```python
from build123d import *

# Parameters (mm, degrees)
SKETCH1_W                 = 14.2875
SKETCH1_H                 = 6.35
EXTRUDE1_DEPTH            = 44.45
F_6_CLEARANCE_HOLE1_D     = 3.7973
F_6_CLEARANCE_HOLE1_DEPTH = 6.35
F_6_CLEARANCE_HOLE1_TIP   = 1.140824014
F_6_CLEARANCE_HOLE2_D     = 3.7973
F_6_CLEARANCE_HOLE2_DEPTH = 6.35
F_6_CLEARANCE_HOLE2_TIP   = 1.140824014


with BuildPart() as part:
    # Sketch1 → Extrude1 (new body)
    with BuildSketch(Plane(origin=(0, 0, 0), x_dir=(1, 0, 0), z_dir=(0, 1, 0))):
        with Locations((-45.973078165, 33.616731266)):
            Rectangle(SKETCH1_W, SKETCH1_H)
    extrude(amount=EXTRUDE1_DEPTH)

    # #6 Clearance Hole1
    with Locations(Plane(origin=(0, 44.45, 0), x_dir=(-1, 0, 0), z_dir=(0, 1, 0))):
        with Locations((45.973078165, -33.616731266)):
            Hole(F_6_CLEARANCE_HOLE1_D / 2, depth=F_6_CLEARANCE_HOLE1_DEPTH)
            with Locations((0, 0, -(F_6_CLEARANCE_HOLE1_DEPTH + F_6_CLEARANCE_HOLE1_TIP / 2))):  # 118° drill point
                Cone(0, F_6_CLEARANCE_HOLE1_D / 2, F_6_CLEARANCE_HOLE1_TIP, mode=Mode.SUBTRACT)

    # #6 Clearance Hole2
    with Locations(Plane(origin=(-45.973078165, 0, -33.616731266), x_dir=(0, 0, -1), z_dir=(0, -1, 0))):
        with Locations((0, 0)):
            Hole(F_6_CLEARANCE_HOLE2_D / 2, depth=F_6_CLEARANCE_HOLE2_DEPTH)
            with Locations((0, 0, -(F_6_CLEARANCE_HOLE2_DEPTH + F_6_CLEARANCE_HOLE2_TIP / 2))):  # 118° drill point
                Cone(0, F_6_CLEARANCE_HOLE2_D / 2, F_6_CLEARANCE_HOLE2_TIP, mode=Mode.SUBTRACT)


solid = part.part
```
Source: CAD feature listing. Evaluate the final solid. Frame: model axes, mm. A direction names the side the tool comes from. Give positions to 0.01 mm unless a question says otherwise; leave off trailing zeros. Loops run counter-clockwise (first coordinate to the right, second up) from the corner with the lowest first, then second, coordinate; pieces in that order, holes last. Notation, with made-up numbers: (60, -38) -> (91, -38) arc R16 cw to (91, -33) -> close; hole circle Ø9 at (-13.5, 29.25). An arc over 180 degrees is marked (long way). Use a Markdown table: item, result. Add a question column.
(1) Section query A-A (y = 41). Output: boundary loops of the cut face in (x, z).
(2) Access query for faces 1 (the face through (-47.37, 41.23, -32.33)), 2 (the face through (-45.403, 3.219, -31.806)), 3 (the face through (-46.1, 0, -31.5)). Directions: +Z, -Z, +X, -X, +Y, -Y. A direction counts if a zero-diameter tool reaches every point of the face in a straight line with its end or side. Return the directions, or none.
(3) Pull-direction query (Z, two-part tool) for faces 4 (the face through (-46.1, 44.45, -31.5)), 5 (the face through (-46.13, 37.16, -33.91)), 6 (the face through (-45.646, 7.293, -33.574)), 7 (the face through (-46, 22, -30.442)); classes: +Z half, -Z half, draft (parallel to the pull), parting line (faces both ways), or undercut.
(4) Ray query, line 1 (Z direction, x = -46, y = 38.5); line 2 (Z direction, x = -45, y = 39); line 3 (X direction, y = 39.5, z = -32.25). Return the intervals inside material, ascending.
(5) First-contact query: pin 1 Ø2.5 at (x, z) = (-45.97, -33.62) entering from +Y; pin 2 Ø3.5 at (x, z) = (-45.97, -33.62) entering from +Y. Flat tips, straight axial feed; report the tip coordinate or a pass-through.
Checked values:
| question | item | result |
|---|---|---|
| 1 | outline | (-53.12, -36.79) -> (-38.83, -36.79) -> (-38.83, -30.44) -> (-53.12, -30.44) -> close; hole circle Ø3.8 at (-45.97, -33.62) |
| 2 | face 1 | +Y |
| 2 | face 2 | -Y |
| 2 | face 3 | +Z, -Z, +X, -X, -Y |
| 3 | face 4 | draft |
| 3 | face 5 | undercut |
| 3 | face 6 | undercut |
| 3 | face 7 | +Z half |
| 4 | line 1 | -36.79 to -35.52, -31.72 to -30.44 |
| 4 | line 2 | -36.79 to -35.25, -31.99 to -30.44 |
| 4 | line 3 | -53.12 to -47.29, -44.66 to -38.83 |
| 5 | pin 1 | y = 37.71 |
| 5 | pin 2 | y = 38.01 |
